Geometry: final body of the model. Coordinates: model frame, mm. Give positions to 0.01 mm unless a question says otherwise; leave off trailing zeros. Loops run counter-clockwise (first coordinate to the right, second up) from the corner with the lowest first, then second, coordinate; pieces in that order, holes last. Notation, with made-up numbers: (58, 71.5) -> (109, 71.5) arc R26 cw to (109, 98.5) -> close; hole circle Ø9 at (-20, -1). An arc over 180 degrees is marked (long way). One line per question, with ' | ' between items. Start each with the question number.
Item 1: Section A-A on x = 33. Return loops of the section in (y, z).
Item 2: Pin query (flat end, axial travel): P1, Ø0.8, axis at x = -17, z = 2, coming from the +Y side; P2, Ø1.5, axis at x = -16, z = 1, coming from the -Y side. Return the tip coordinate at first contact, or that it passes through.
Item 3: Material intervals for line 1 along X through (y, z) = (17.5, 1.05); line 2 along Y through (x, z) = (14.5, 0.7); line 3 along X through (y, z) = (44.5, 2.65), sorted ascending. Write a range as [from, to].
Item 4: Section B-B on y = 25. Return loops of the section in (x, z), then the cut area to 3 significant figures.
from build123d import *

# Parameters (mm, degrees)
SKETCH1_W           = 80.3
SKETCH1_H           = 66
BOSS_EXTRUDE1_DEPTH = 3
FILLET1_R           = 3.5
SKETCH2_W           = 72.4
SKETCH2_H           = 45
CUT_EXTRUDE1_DEPTH  = 4
SKETCH3_W           = 15
SKETCH3_H           = 30
SKETCH3_W_2         = 33
SKETCH3_H_2         = 18
SKETCH3_W_3         = 39
SKETCH3_H_3         = 18.5
CUT_EXTRUDE2_DEPTH  = 4
SKETCH4_W           = 39
SKETCH4_H           = 18.5
SKETCH4_W_2         = 15
SKETCH4_H_2         = 30
SKETCH4_W_3         = 72.4
SKETCH4_H_3         = 45
CUT_EXTRUDE3_DEPTH  = 4


with BuildPart() as part:
    # Sketch1 → Boss-Extrude1 (new body)
    with BuildSketch(Plane.XY):
        Polygon((-18, -20), (60.3, -20), (80.3, 0), (0, 0), (0, 66), (-18, 48), align=None)
        with Locations((40.15, 33)):
            Rectangle(SKETCH1_W, SKETCH1_H)
    extrude(amount=BOSS_EXTRUDE1_DEPTH)

    # Fillet1
    fillet1_edges = [part.edges().sort_by_distance(p)[0] for p in [
        (60.3, -20, 1.5),
        (-18, -20, 1.5),
        (-18, 48, 1.5),
        (0, 66, 1.5),
        (80.3, 66, 1.5),
        (80.3, 0, 1.5),
    ]]
    fillet(fillet1_edges, radius=FILLET1_R)

    # Sketch2 → Cut-Extrude1 (cut, through all)
    with BuildSketch(Plane.XY.offset(3)):
        with Locations((39.2, 33)):
            Rectangle(SKETCH2_W, SKETCH2_H)
    extrude(amount=-CUT_EXTRUDE1_DEPTH, mode=Mode.SUBTRACT)

    # Sketch3 → Cut-Extrude2 (cut, through all)
    with BuildSketch(Plane.XY.offset(3)):
        with BuildLine():
            Line((-3, 47.3), (-17.918753974, 47.3))
            ThreePointArc((-17.918753974, 47.3), (-17.979629212, 46.927320889), (-18, 46.550252532))
            Line((-18, 46.550252532), (-18, 36.5))
            Line((-18, 36.5), (-3, 36.5))
            Line((-3, 36.5), (-3, 47.3))
        make_face()
        with Locations((-7.5, 19.5)):
            Rectangle(SKETCH3_W, SKETCH3_H)
        with Locations((43.5, -8)):
            Rectangle(SKETCH3_W_2, SKETCH3_H_2)
        with Locations((4.5, -7.75)):
            Rectangle(SKETCH3_W_3, SKETCH3_H_3)
        Polygon((67.242640687, -0.329437252), (63, -4.572077939), (67.242640687, -8.814718626), (71.485281374, -4.572077939), align=None)
    extrude(amount=-CUT_EXTRUDE2_DEPTH, mode=Mode.SUBTRACT)

    # Sketch4 → Cut-Extrude3 (cut, through all)
    with BuildSketch(Plane.XY.offset(3)):
        with BuildLine():
            Line((0.919417382, 63.030330086), (-14.810912703, 47.3))
            Line((-14.810912703, 47.3), (-3, 47.3))
            Line((-3, 47.3), (-3, 36.5))
            Line((-3, 36.5), (-15.249922187, 36.5))
            Line((-15.249922187, 36.5), (-15.25, 36.489656324))
            Line((-15.25, 36.489656324), (-15.25, -16.5))
            ThreePointArc((-15.25, -16.5), (-15.030330086, -17.030330086), (-14.5, -17.25))
            Line((-14.5, -17.25), (58.850252532, -17.25))
            ThreePointArc((58.850252532, -17.25), (59.137265106, -17.192909649), (59.380582618, -17.030330086))
            Line((59.380582618, -17.030330086), (59.410912703, -17))
            Line((59.410912703, -17), (27, -17))
            Line((27, -17), (27, 1))
            Line((27, 1), (60, 1))
            Line((60, 1), (60, -16.410912703))
            Line((60, -16.410912703), (77.330330086, 0.919417382))
            ThreePointArc((77.330330086, 0.919417382), (77.492909649, 1.162734894), (77.55, 1.449747468))
            Line((77.55, 1.449747468), (77.55, 62.5))
            ThreePointArc((77.55, 62.5), (77.330330086, 63.030330086), (76.8, 63.25))
            Line((76.8, 63.25), (1.449747468, 63.25))
            ThreePointArc((1.449747468, 63.25), (1.162734894, 63.192909649), (0.919417382, 63.030330086))
        make_face()
        with Locations((4.5, -7.75)):
            Rectangle(SKETCH4_W, SKETCH4_H, mode=Mode.SUBTRACT)
        with Locations((-7.5, 19.5)):
            Rectangle(SKETCH4_W_2, SKETCH4_H_2, mode=Mode.SUBTRACT)
        Polygon((67.242640687, -8.814718626), (63, -4.572077939), (67.242640687, -0.329437252), (71.485281374, -4.572077939), align=None, mode=Mode.SUBTRACT)
        with Locations((39.2, 33)):
            Rectangle(SKETCH4_W_3, SKETCH4_H_3, mode=Mode.SUBTRACT)
    extrude(amount=-CUT_EXTRUDE3_DEPTH, mode=Mode.SUBTRACT)


solid = part.part
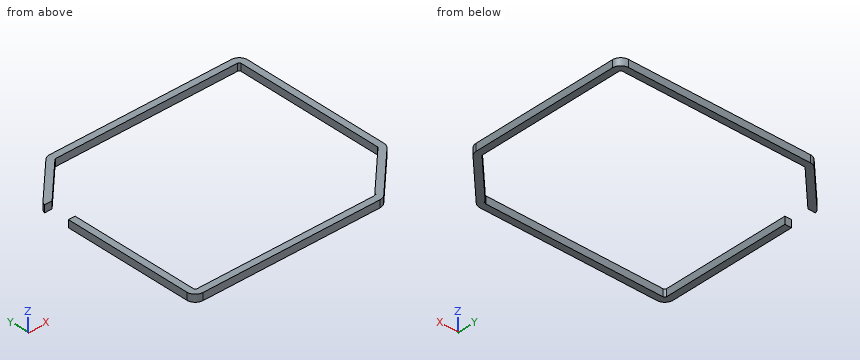
Result sheet:
1) outline: (-20, 0) -> (-17.25, 0) -> (-17.25, 3) -> (-20, 3) -> close; (63.25, 0) -> (66, 0) -> (66, 3) -> (63.25, 3) -> close
2) P1: stops at y = 49.4 | P2: stops at y = -19.92
3) line 1: x = [-18, -15.25], [77.55, 80.3] | line 2: y = [-20, -17.25], [63.25, 66] | line 3: x = [77.55, 80.3]
4) outline: (-18, 0) -> (-15.25, 0) -> (-15.25, 3) -> (-18, 3) -> close; (77.55, 0) -> (80.3, 0) -> (80.3, 3) -> (77.55, 3) -> close | area: 16.5 mm²
